from build123d import *

# Parameters (mm, degrees)
SKETCH1_W                       = 13.5
SKETCH1_H                       = 20
BOSS_EXTRUDE1_DEPTH             = 22.7
SKETCH2_W                       = 50.012416784
SKETCH2_H                       = 57.752903126
CUT_EXTRUDE1_DEPTH              = 22.813888303
M2X0_4_TAPPED_HOLE1_D           = 1.6
M2X0_4_TAPPED_HOLE1_ON_FACE_2_D = 1.6
M2X0_4_TAPPED_HOLE1_ON_FACE_3_D = 1.6
M2X0_4_TAPPED_HOLE3_D           = 1.6
F_1_0MM_DOWEL_HOLE1_D           = 1
F_1_5MM_DOWEL_HOLE1_D           = 1.5
F_1_5MM_DOWEL_HOLE1_DEPTH       = 4.5
F_1_5MM_DOWEL_HOLE1_TIP         = 0.450645464
F_1_0MM_DOWEL_HOLE2_D           = 1
F_1_0MM_DOWEL_HOLE2_ON_FACE_2_D = 1
F_1_5MM_DOWEL_HOLE2_D           = 1.5
F_1_5MM_DOWEL_HOLE2_DEPTH       = 3.5
F_1_5MM_DOWEL_HOLE2_TIP         = 0.450645464


with BuildPart() as part:
    # Sketch1 → Boss-Extrude1 (new body)
    with BuildSketch(Plane(origin=(0, 0, 0), x_dir=(1, 0, 0), z_dir=(0, 1, 0))):
        with Locations((6.75, 10)):
            Rectangle(SKETCH1_W, SKETCH1_H)
    extrude(amount=BOSS_EXTRUDE1_DEPTH)

    # Sketch2 → Cut-Extrude1 (cut, through all)
    with BuildSketch(Plane(origin=(7.815425957, 6.381268572, -7.815425957), x_dir=(0.7905694150420965, -0.3872983346207431, 0.4743416490252531), z_dir=(-0.6123724356957925, -0.5000000000000046, 0.6123724356957929))):
        Rectangle(SKETCH2_W, SKETCH2_H)
    extrude(amount=-CUT_EXTRUDE1_DEPTH, mode=Mode.SUBTRACT)

    # M2x0.4 Tapped Hole1 (through all)
    with Locations(Plane(origin=(6.5161982, 14.294607438, -2.653439586), x_dir=(-0.707106781187, 0, -0.707106781187), z_dir=(0.612372435696, 0.5, -0.612372435696))):
        with Locations((0, 0)):
            Hole(M2X0_4_TAPPED_HOLE1_D / 2)

    # M2x0.4 Tapped Hole1 on face 2 (through all)
    with Locations(Plane(origin=(8.855545244, 8.665670048, -4.910100675), x_dir=(-0.707106781187, 0, -0.707106781187), z_dir=(0.612372326772, 0.500000266808, -0.612372326772))):
        with Locations((0, 0)):
            Hole(M2X0_4_TAPPED_HOLE1_ON_FACE_2_D / 2)

    # M2x0.4 Tapped Hole1 on face 3 (through all)
    with Locations(Plane(origin=(5.007385282, 2.349364905, -13.91550219), x_dir=(-0.707106781187, 0, -0.707106781187), z_dir=(0.612372326772, 0.500000266808, -0.612372326772))):
        with Locations((0, 0)):
            Hole(M2X0_4_TAPPED_HOLE1_ON_FACE_3_D / 2)

    # M2x0.4 Tapped Hole3 (through all)
    with Locations(Plane(origin=(1.5, 16, 0), x_dir=(1, 0, 0), z_dir=(0, 0, 1))):
        with Locations((0, 0), (0, -14), (9, -14)):
            Hole(M2X0_4_TAPPED_HOLE3_D / 2)

    # Ø1.0mm Dowel Hole1 (through all)
    with Locations(Plane(origin=(5.5, 10, 0), x_dir=(1, 0, 0), z_dir=(0, 0, 1))):
        with Locations((0, 0), (4, -4)):
            Hole(F_1_0MM_DOWEL_HOLE1_D / 2)

    # Ø1.5mm Dowel Hole1
    with Locations(Plane(origin=(5.5, 10, 0), x_dir=(1, 0, 0), z_dir=(0, 0, 1))):
        with Locations((0, 0), (4, -4)):
            Hole(F_1_5MM_DOWEL_HOLE1_D / 2, depth=F_1_5MM_DOWEL_HOLE1_DEPTH)
            with Locations((0, 0, -(F_1_5MM_DOWEL_HOLE1_DEPTH + F_1_5MM_DOWEL_HOLE1_TIP / 2))):  # 118° drill point
                Cone(0, F_1_5MM_DOWEL_HOLE1_D / 2, F_1_5MM_DOWEL_HOLE1_TIP, mode=Mode.SUBTRACT)

    # Ø1.0mm Dowel Hole2 (through all)
    with Locations(Plane(origin=(3.59317172, 12.741669751, -6.844434378), x_dir=(-0.707106781187, 0, -0.707106781187), z_dir=(0.612372435696, 0.5, -0.612372435696))):
        with Locations((0, 0)):
            Hole(F_1_0MM_DOWEL_HOLE2_D / 2)

    # Ø1.0mm Dowel Hole2 on face 2 (through all)
    with Locations(Plane(origin=(7.128705626, 4.081415713, -10.379968284), x_dir=(-0.707106781187, 0, -0.707106781187), z_dir=(0.612372326772, 0.500000266808, -0.612372326772))):
        with Locations((0, 0)):
            Hole(F_1_0MM_DOWEL_HOLE2_ON_FACE_2_D / 2)

    # Ø1.5mm Dowel Hole2
    with Locations(Plane(origin=(3.59317172, 12.741669751, -6.844434378), x_dir=(-0.707106781187, 0, -0.707106781187), z_dir=(0.612372435696, 0.5, -0.612372435696))):
        with Locations((0, 0), (0, -10)):
            Hole(F_1_5MM_DOWEL_HOLE2_D / 2, depth=F_1_5MM_DOWEL_HOLE2_DEPTH)
            with Locations((0, 0, -(F_1_5MM_DOWEL_HOLE2_DEPTH + F_1_5MM_DOWEL_HOLE2_TIP / 2))):  # 118° drill point
                Cone(0, F_1_5MM_DOWEL_HOLE2_D / 2, F_1_5MM_DOWEL_HOLE2_TIP, mode=Mode.SUBTRACT)


solid = part.part
Model file for the job. Use its own axes, mm. A direction names the side the tool comes from. Round coordinates to 2 decimals unless told otherwise and drop trailing zeros. Loops run counter-clockwise (first coordinate to the right, second up) from the corner with the lowest first, then second, coordinate; pieces in that order, holes last. Notation, with made-up numbers: M -6.75,-9.75 L 7.25,-9.75 A23 cw 7.25,13.25 Z; hole C -36.5,88.5 d5. An arc over 180 degrees is marked long. One line per question, with ' | ' between items.
1) Drill centre lines: line 1 along X through (y, z) = (6, -2.1); line 2 along X through (y, z) = (1.75, -13.5); line 3 along X through (y, z) = (2, -11.5). Where is each one in solid material? Low to high.
Solved:
line 1: x = 0 to 4.92, 6.81 to 8.75, 10.25 to 13.5 | line 2: x = 0 to 0.74, 2.26 to 3.49, 5.44 to 5.91 | line 3: x = 0 to 0.7, 2.3 to 7.71
2) Band-saw the part on A-A (y = 16). Give the cut face in (x, z), then the cut area to 3 significant figures.
Solved:
outline: M 0,-7.78 L 0.7,-7.08 L 0.7,0 L 0,0 Z; M 2.3,-5.48 L 7.78,0 L 2.3,0 Z | area: 20.2 mm²
3) Flat gauge pins, fed straight in: pin 1 (1.5 mm diameter, centred on y = 7, z = -15, fed in from -X); pin 2 (2.5 mm diameter, centred on x = 1.5, y = 16, fed in from -Z); pin 3 (2.5 mm diameter, centred on x = 1.5, y = 2, fed in from -Z); pin 4 (1.5 mm diameter, centred on y = 4.5, z = -8, fed in from +X). Where does each tip first touch, or does it go through?
Solved:
pin 1: stops at x = 0 | pin 2: stops at z = -7.89 | pin 3: stops at z = -19.32 | pin 4: stops at x = 10.14
4) Band-saw the part on C-C (y = 6). Give the number of separate pieces and of enclosed holes in the cut face, then the cut area to 3 significant figures.
Solved:
separate pieces: 2 | enclosed holes: 1 | area: 111 mm²
5) Band-saw the part on B-B (z = -17.75). Give the cut face in (x, y), then the cut area to 3 significant figures.
Solved:
outline: M 0,0 L 3.09,0 L 1.98,1.36 A0.8 cw 0.97,2.6 L 0,3.79 Z | area: 4.90 mm²
6) 3-axis set-ups, long thin cutter, end or side, ignore diameter. For faces 1 (the flat face through (5, 9, 0)), 2 (the cylindrical face through (6.05, 10.51, -2.28)): which of +Z, -Z, +X, -X, +Y, -Y reach the whole face in a straight line?
Solved:
face 1: +Z, +X, -X, +Y, -Y | face 2: +Z
7) Band-saw the part on D-D (x = 12.25). Give the cut face in (y, z), then the cut area to 3 significant figures.
Solved:
outline: M 0,-8.59 L 10.52,0 L 0,0 Z | area: 45.2 mm²
8) Mould opens along X. For faces 3 (the cylindrical face through (2.57, 12.4, -5.25)), 4 (the flat face through (6.655, 9.024, -6.817)), 5 (the flat face through (1, 22.7, -1)) say: +X half, -X half, draft (parallel to the pull), parting line (faces both ways), or undercut.
Solved:
face 3: undercut | face 4: +X half | face 5: draft
